Input: part model. Units: mm. Frame: model coordinates. A direction names the side the tool comes from. Coordinates: 2 decimals unless noted, no trailing zeros. Write each loop counter-clockwise with the first axis right and the second up, starting at its lowest first coordinate (ties: lowest second). Pieces come first, ordered by that corner, then holes.
1) Pin query (flat end, axial travel): pin 1 Ø6 at (x, z) = (4, 2.5) entering from -Y; pin 2 Ø4 at (x, z) = (-4, 0.5) entering from -Y; pin 3 Ø1.1 at (x, y) = (-1.5, -4.5) entering from +Z. Return the tip coordinate at first contact, or that it passes through.
2) Section query A-A (x = 5.25). Output: boundary loops of the cut face in (y, z), then the cut area to 3 significant figures.
3) Line query: L1, parallel to Z at x = -5.75, y = -0.25; L2, parallel to Z at x = 1.5, y = 3.75; L3, parallel to Y at x = -6, z = 1. Output: solid intervals per line, ascending.
4) Set-up query: faces 1 (the flat face through (3, -4, 0)), 2 (the cylindrical face through (-2.78, 5.235, 3.451)), 3 (the cylindrical face through (-4.485, -3.875, 3.451)), 4 (the cylindrical face through (4.78, -3.51, 3.45)). Return all of +Z, -Z, +X, -X, +Y, -Y with unobstructed straight access to the full face (end or side cutting, diameter ignored); none if empty.
5) Draft query along Z for faces 5 (the flat face through (0, 0, -9.5)), 6 (the flat face through (0, 0, -25)), 7 (the cylindrical face through (4.909, 3.368, 3.451)), 8 (the flat face through (-1, 5, 0)). Return one class per face: pulls with the +Z half, pulls with the -Z half, needs draft (parallel to the pull), parting line crosses it, or undercut.
6) Section query B-B (x = -5.5). Output: boundary loops of the cut face in (y, z).
from build123d import *

# Parameters (mm, degrees)
SKETCH2_R                   = 6.75
GEAR_OUTSIDE_DIAMETER_DEPTH = 7
GEAR_TOOTH_CUT_DEPTH        = 8
GEAR_TEETH_COUNT            = 7
SKETCH3_R                   = 3.375
GEAR_DEDENDUM_CIRCLE_DEPTH  = 7
SKETCH8_R                   = 2.7
BOSS_EXTRUDE3_DEPTH         = 9.5
BOSS_EXTRUDE2_DEPTH         = 15.5
BOSS_EXTRUDE2_TAPER         = 0.5
SKETCH9_R                   = 6.75
BOSS_EXTRUDE4_DEPTH         = 0.4


with BuildPart() as part:
    # Sketch2 → gear outside diameter (new body)
    with BuildSketch(Plane.XY):
        Circle(SKETCH2_R)
    extrude(amount=GEAR_OUTSIDE_DIAMETER_DEPTH)

    # Sketch1 → gear tooth cut (cut, through all)
    with BuildSketch(Plane.XY):
        with BuildLine():
            Line((0, 4.933386259), (0, 3.375))
            ThreePointArc((0, 3.375), (-0.701885443, 3.301209146), (-1.373078899, 3.083063304))
            Line((-1.373078899, 3.083063304), (-2.007089948, 4.506649523))
            ThreePointArc((-2.007089948, 4.506649523), (-2.793182164, 5.242332608), (-3.820403893, 5.564801352))
            ThreePointArc((-3.820403893, 5.564801352), (-1.403770885, 6.602418292), (1.225966143, 6.637733575))
            ThreePointArc((1.225966143, 6.637733575), (0.41879145, 5.925245269), (0, 4.933386259))
        make_face()
    gear_tooth_cut = extrude(amount=GEAR_TOOTH_CUT_DEPTH, mode=Mode.SUBTRACT)

    # gear teeth: gear tooth cut ×7 about axis
    gear_teeth_axis = Axis((0, 0, 0), (0, 0, 1))
    for i in range(1, GEAR_TEETH_COUNT):
        add(gear_tooth_cut.rotate(gear_teeth_axis, i * 360 / GEAR_TEETH_COUNT), mode=Mode.SUBTRACT)

    # Sketch3 → gear dedendum circle (add)
    with BuildSketch(Plane.XY):
        Circle(SKETCH3_R)
    extrude(amount=GEAR_DEDENDUM_CIRCLE_DEPTH)

    # Sketch8 → Boss-Extrude3 (add)
    with BuildSketch(Plane(origin=(0, 0, 0), x_dir=(-1, 0, 0), z_dir=(0, 0, -1))):
        with Locations((-2.068006907, 3.746919537)):
            Circle(SKETCH8_R)
    extrude(amount=BOSS_EXTRUDE3_DEPTH)

    # Sketch6 → Boss-Extrude2 (add)
    with BuildSketch(Plane(origin=(0, 0, -9.5), x_dir=(-1, 0, 0), z_dir=(0, 0, -1))):
        with BuildLine():
            ThreePointArc((1.6, 0.824621125), (0, 1.8), (-1.6, 0.824621125))
            Line((-1.6, 0.824621125), (-1.6, -0.824621125))
            ThreePointArc((-1.6, -0.824621125), (0, -1.8), (1.6, -0.824621125))
            Line((1.6, -0.824621125), (1.6, -0.6))
            Line((1.6, -0.6), (1.697056275, -0.6))
            Line((1.697056275, -0.6), (1.697056275, 0.6))
            Line((1.697056275, 0.6), (1.6, 0.6))
            Line((1.6, 0.6), (1.6, 0.824621125))
        make_face()
    extrude(amount=BOSS_EXTRUDE2_DEPTH, taper=BOSS_EXTRUDE2_TAPER)

    # Sketch9 → Boss-Extrude4 (add)
    with BuildSketch(Plane(origin=(0, 0, 0), x_dir=(-1, 0, 0), z_dir=(0, 0, -1))):
        Circle(SKETCH9_R)
    extrude(amount=BOSS_EXTRUDE4_DEPTH)


solid = part.part
Answer:
1. pin 1: stops at y = -6.67
1. pin 2: stops at y = -6.43
1. pin 3: stops at z = 0
2. outline: (-4.24, -0.4) - (4.24, -0.4) - (4.24, 0) - (3.36, 0) - (3.36, 7) - (1.16, 7) - (1.16, 0) - (-1.34, 0) - (-1.34, 7) - (-3.5, 7) - (-3.5, 0) - (-4.24, 0) - close
2. area: 33.9 mm2
3. L1: z = -0.4 to 7
3. L2: z = -9.5 to 7
3. L3: y = -0.85 to 1.02
4. face 1: +Z
4. face 2: +Z, +Y
4. face 3: +Z, -X
4. face 4: +Z, -Y
5. face 5: undercut
5. face 6: pulls with the -Z half
5. face 7: needs draft
5. face 8: pulls with the +Z half
6. outline: (-3.91, -0.4) - (3.91, -0.4) - (3.91, 0) - (1.19, 0) - (1.19, 7) - (-1.03, 7) - (-1.03, 0) - (-3.91, 0) - close
